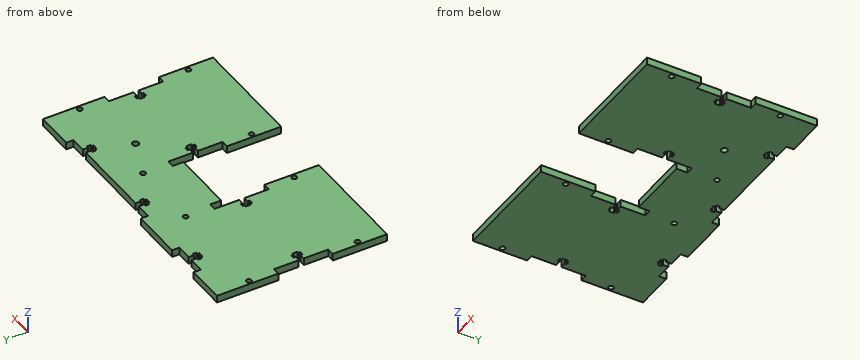
from build123d import *

# Parameters (mm, degrees)
SKETCH_1_R      = 1.4
SKETCH_1_R_2    = 1.75
EXTRUDE_1_DEPTH = 4


with BuildPart() as part:
    # Эскиз1 → Бобышка-Вытянуть1 (new body)
    with BuildSketch(Plane.XY):
        Polygon((-17.5, -14), (-17.5, -20), (17.5, -20), (17.5, -14), (21.5, -14), (21.5, -27.6), (24.5, -27.6), (24.5, -26.45), (26.5, -26.45), (26.5, -27.6), (27.5, -27.6), (27.5, -30.4), (26.5, -30.4), (26.5, -31.55), (24.5, -31.55), (24.5, -30.4), (21.5, -30.4), (21.5, -44), (17.5, -44), (17.5, -74), (80.5, -74), (80.5, -44), (76.5, -44), (76.5, -30.4), (73.5, -30.4), (73.5, -31.55), (71.5, -31.55), (71.5, -30.4), (70.5, -30.4), (70.5, -27.6), (71.5, -27.6), (71.5, -26.45), (73.5, -26.45), (73.5, -27.6), (76.5, -27.6), (76.5, -14), (80.5, -14), (80.5, 20), (59, 20), (59, 16), (50.4, 16), (50.4, 13), (51.55, 13), (51.55, 11), (50.4, 11), (50.4, 10), (47.6, 10), (47.6, 11), (46.45, 11), (46.45, 13), (47.6, 13), (47.6, 16), (1.4, 16), (1.4, 13), (2.55, 13), (2.55, 11), (1.4, 11), (1.4, 10), (-1.4, 10), (-1.4, 11), (-2.55, 11), (-2.55, 13), (-1.4, 13), (-1.4, 16), (-10, 16), (-10, 20), (-39, 20), (-39, 16), (-47.6, 16), (-47.6, 13), (-46.45, 13), (-46.45, 11), (-47.6, 11), (-47.6, 10), (-50.4, 10), (-50.4, 11), (-51.55, 11), (-51.55, 13), (-50.4, 13), (-50.4, 16), (-59, 16), (-59, 20), (-80.5, 20), (-80.5, -14), (-76.5, -14), (-76.5, -27.6), (-73.5, -27.6), (-73.5, -26.45), (-71.5, -26.45), (-71.5, -27.6), (-70.5, -27.6), (-70.5, -30.4), (-71.5, -30.4), (-71.5, -31.55), (-73.5, -31.55), (-73.5, -30.4), (-76.5, -30.4), (-76.5, -44), (-80.5, -44), (-80.5, -74), (-17.5, -74), (-17.5, -44), (-21.5, -44), (-21.5, -30.4), (-24.5, -30.4), (-24.5, -31.55), (-26.5, -31.55), (-26.5, -30.4), (-27.5, -30.4), (-27.5, -27.6), (-26.5, -27.6), (-26.5, -26.45), (-24.5, -26.45), (-24.5, -27.6), (-21.5, -27.6), (-21.5, -14), align=None)
        with Locations((-19.75, 1)):
            Circle(SKETCH_1_R, mode=Mode.SUBTRACT)
        with Locations((-78.25, -59)):
            Circle(SKETCH_1_R, mode=Mode.SUBTRACT)
        with Locations((-19.75, -59)):
            Circle(SKETCH_1_R, mode=Mode.SUBTRACT)
        with Locations((-78.25, 1)):
            Circle(SKETCH_1_R, mode=Mode.SUBTRACT)
        with Locations((78.25, 1)):
            Circle(SKETCH_1_R, mode=Mode.SUBTRACT)
        with Locations((19.75, -59)):
            Circle(SKETCH_1_R, mode=Mode.SUBTRACT)
        with Locations((78.25, -59)):
            Circle(SKETCH_1_R, mode=Mode.SUBTRACT)
        with Locations((41.5, -7.9)):
            Circle(SKETCH_1_R_2, mode=Mode.SUBTRACT)
        with Locations((19.75, 1)):
            Circle(SKETCH_1_R, mode=Mode.SUBTRACT)
    extrude(amount=EXTRUDE_1_DEPTH)


solid = part.part
Verification items for the finished model (mm, model axes). Coordinates: 2 decimals unless noted, no trailing zeros. Order: outer loops, then holes, each group sorted by start corner. A loop starts at its lowest first (then second) coordinate and runs counter-clockwise, first axis right, second up. Notation, with made-up numbers: (48.25, -30) -> (66.25, -30) arc R30 ccw to (66.25, -8) -> close; hole circle Ø4 at (36.25, 14.25). An arc over 180 degrees is marked (long way). Use CSV: the item, a comma, the result in double quotes. Start each with the question number.
Q1. Section check C-C, the plane z = 1.3. Give the number of separate pieces and of enclosed holes in the cut face, and give its area (3 significant figures).
Q2. Section check D-D, the plane x = 12. Record the cut outline in (y, z), and give its area (3 significant figures).
Q3. Section check A-A, the plane x = 41.5. Record the cut outline in (y, z).
Q4. Section check B-B, the plane y = -52. Record the cut outline in (x, z), and give its area (3 significant figures).
Q5. Depth check by flat-ended pin: P1, Ø0.6, axis at x = 51, z = 2.5, coming from the +Y side; P2, Ø1.2, axis at y = -34.5, z = 1.5, coming from the -X side; P3, Ø0.6, axis at y = -31, z = 2.5, coming from the +X side. Enter the tip coordinate at first touch or a pass-through.
Q6. Thickness scan on line 1 along Y through (x, z) = (-78.25, 3.2); line 2 along X through (y, z) = (-41.5, 0.7); line 3 along X through (y, z) = (-64.5, 3.2). Record the ranges inside material, lowest first.
Returned:
1,separate pieces,"1"
1,enclosed holes,"9"
1,area,"12,200 mm^2"
2,outline,"(-20, 0) -> (16, 0) -> (16, 4) -> (-20, 4) -> close"
2,area,"144 mm^2"
3,outline,"(-74, 0) -> (-9.65, 0) -> (-9.65, 4) -> (-74, 4) -> close; (-6.15, 0) -> (16, 0) -> (16, 4) -> (-6.15, 4) -> close"
4,outline,"(-80.5, 0) -> (-17.5, 0) -> (-17.5, 4) -> (-80.5, 4) -> close; (17.5, 0) -> (80.5, 0) -> (80.5, 4) -> (17.5, 4) -> close"
4,area,"504 mm^2"
5,P1,"stops at y = 16"
5,P2,"stops at x = -76.5"
5,P3,"stops at x = 76.5"
6,line 1,"y = -74 to -60.4, -57.6 to -44, -14 to -0.4, 2.4 to 20"
6,line 2,"x = -76.5 to -21.5, 21.5 to 76.5"
6,line 3,"x = -80.5 to -17.5, 17.5 to 80.5"
